from build123d import *

# Parameters (mm, degrees)
SALIENTE_EXTRUIR2_DEPTH      = 30.5
CROQUIS14_R                  = 25.5
CORTAR_EXTRUIR1_DEPTH        = 12
SALIENTE_EXTRUIR3_DEPTH      = 30
SALIENTE_EXTRUIR3_DEPTH_BACK = 4
CROQUIS15_R                  = 14
CROQUIS16_R                  = 11.5
CORTAR_EXTRUIR2_DEPTH        = 25
SKETCH1_W                    = 18
SKETCH1_H                    = 53
CUT_EXTRUDE1_DEPTH           = 8.5
SKETCH2_R                    = 4
CUT_EXTRUDE2_DEPTH           = 3
SKETCH3_R                    = 2.45
BOSS_EXTRUDE1_DEPTH          = 8.5
SKETCH4_W                    = 2.6
SKETCH4_H                    = 5
BOSS_EXTRUDE2_DEPTH          = 12.4


with BuildPart() as part:
    # Croquis13 → Saliente-Extruir2 (new body)
    with BuildSketch(Plane.XY):
        with BuildLine():
            Line((63.278452832, -47.557716663), (115.634697867, -47.557716663))
            add(Edge.make_bspline(
                [(115.634697867, -47.557716663), (120.956575349, -31.401681318), (120.956575349, -11.961207195)],
                knots=[0.980995561, 0.980995561, 0.980995561, 1.570796327, 1.570796327, 1.570796327], degree=2, weights=[1, 0.9568311, 1]))
            ThreePointArc((120.956575349, -11.961207195), (89.456575349, 19.538792805), (57.956575349, -11.961207195))
            add(Edge.make_bspline(
                [(57.956575349, -11.961207195), (57.956575349, -31.401681318), (63.278452832, -47.557716663)],
                knots=[4.71238898, 4.71238898, 4.71238898, 5.302189747, 5.302189747, 5.302189747], degree=2, weights=[1, 0.9568311, 1]))
        make_face()
    extrude(amount=SALIENTE_EXTRUIR2_DEPTH)

    # Croquis14 → Cortar-Extruir1 (cut)
    with BuildSketch(Plane.XY.offset(30.5)):
        with Locations((89.456575349, -11.961207195)):
            Circle(CROQUIS14_R)
        with BuildLine():
            add(Edge.make_bspline(
                [(109.141957532, -47.557716663), (114.956575349, -32.049805489), (114.956575349, -11.961207195)],
                knots=[4.023536226, 4.023536226, 4.023536226, 4.71238898, 4.71238898, 4.71238898], degree=2, weights=[1, 0.941269295, 1]))
            ThreePointArc((114.956575349, -11.961207195), (89.456575349, -37.461207195), (63.956575349, -11.961207195))
            add(Edge.make_bspline(
                [(63.956575349, -11.961207195), (63.956575349, -32.049805489), (69.771193166, -47.557716663)],
                knots=[1.570796327, 1.570796327, 1.570796327, 2.259649081, 2.259649081, 2.259649081], degree=2, weights=[1, 0.941269295, 1]))
            Line((69.771193166, -47.557716663), (109.141957532, -47.557716663))
        make_face()
    extrude(amount=-CORTAR_EXTRUIR1_DEPTH, mode=Mode.SUBTRACT)

    # Croquis15 → Saliente-Extruir3 (add, two sides: drawn at the far end of the back side and taken through both)
    with BuildSketch(Plane(origin=(89.456575349, 19.538792805, 30.5), x_dir=(1, 0, 0), z_dir=(0, 1, 0)).offset(-SALIENTE_EXTRUIR3_DEPTH_BACK)):
        with Locations(Location((0, 15.25, 0), (0, 0, 270))):
            Circle(CROQUIS15_R)
    extrude(amount=SALIENTE_EXTRUIR3_DEPTH + SALIENTE_EXTRUIR3_DEPTH_BACK)

    # Croquis16 → Cortar-Extruir2 (cut)
    with BuildSketch(Plane(origin=(0, 49.538792805, 0), x_dir=(1, 0, 0), z_dir=(0, 1, 0))):
        with Locations(Location((89.456575349, -15.25, 0), (0, 0, 270))):
            Circle(CROQUIS16_R)
    extrude(amount=-CORTAR_EXTRUIR2_DEPTH, mode=Mode.SUBTRACT)

    # Sketch1 → Cut-Extrude1 (cut)
    with BuildSketch(Plane(origin=(0, -29.057716663, 18.5), x_dir=(-1, 0, 0), z_dir=(0, 0, -1))):
        with Locations((-88.956575349, 11)):
            Rectangle(SKETCH1_W, SKETCH1_H)
    extrude(amount=CUT_EXTRUDE1_DEPTH, mode=Mode.SUBTRACT)

    # Sketch2 → Cut-Extrude2 (cut)
    with BuildSketch(Plane.XZ.offset(44.557716663)):
        with Locations((88.956575349, 18.5)):
            Circle(SKETCH2_R)
    extrude(amount=CUT_EXTRUDE2_DEPTH, mode=Mode.SUBTRACT)

    # Sketch3 → Boss-Extrude1 (add)
    with BuildSketch(Plane.XY.offset(18.5)):
        with Locations((104.956575349, -32.557716663)):
            Circle(SKETCH3_R)
        with Locations((104.956575349, -2.557716663)):
            Circle(SKETCH3_R)
        with Locations((70.956575349, -17.557716663)):
            Circle(SKETCH3_R)
        with Locations((106.956575349, -17.557716663)):
            Circle(SKETCH3_R)
        with Locations((72.956575349, -32.557716663)):
            Circle(SKETCH3_R)
        with Locations((72.956575349, -2.557716663)):
            Circle(SKETCH3_R)
    extrude(amount=BOSS_EXTRUDE1_DEPTH)

    # Sketch4 → Boss-Extrude2 (add)
    with BuildSketch(Plane.XY.offset(10)):
        with Locations((81.256575349, -8.257716663)):
            Rectangle(SKETCH4_W, SKETCH4_H)
        with Locations((96.656575349, -8.257716663)):
            Rectangle(SKETCH4_W, SKETCH4_H)
    extrude(amount=BOSS_EXTRUDE2_DEPTH)


solid = part.part
Source: CAD feature listing. Evaluate the final solid. Frame: model axes, mm. A direction names the side the tool comes from. Coordinates: 2 decimals unless noted, no trailing zeros. Loops run counter-clockwise (first coordinate to the right, second up) from the corner with the lowest first, then second, coordinate; pieces in that order, holes last. Notation, with made-up numbers: (80, -6) -> (90, -6) arc R31 cw to (90, 30) -> close; hole circle Ø10 at (19.5, 65.5). An arc over 180 degrees is marked (long way). Answer in a Markdown table with one row per item. Add a question column.
Q1. Section D-D on y = 26.5. Return the cut outline in (x, z).
Q2. Section B-B on z = 24. Give the number of separate pieces and of enclosed holes in the cut face, and give its area (3 significant figures).
Q3. Section A-A on x = 87.5. Return the cut outline in (y, z), and give its area (3 significant figures).
Q4. Section C-C on y = 4.5. Return the cut outline in (x, z).
Q5. Pull-direction query (Y, two-part tool) for faces 5 (the face through (100.878, 17.395, 4.87)), 6 (the face through (100.86, 37.21, 13.75)), 7 (the face through (89, -18, 10)), 8 (the face through (82.557, -8, 16)); classes: pulls with the +Y half, pulls with the -Y half, needs draft (parallel to the pull), parting line crosses it, or undercut.
Q6. Ray query, line 1 along Y through (x, z) = (82, 11); line 2 along X through (y, z) = (32.75, 15.25); line 3 along X through (y, z) = (-13, 21.5). Return the intervals inside material, ascending.
Q7. Contact query for flat-ended pins moving along their axis: pin 1 Ø4 at (x, y) = (86.5, 6) entering from +Z; pin 2 Ø2 at (x, y) = (97.5, -8.5) entering from +Z; pin 3 Ø4 at (y, z) = (36.5, 10) entering from -X; pin 4 Ø1.5 at (x, y) = (74, 14.5) entering from -Z. Output: stop coordinate, or through.
Q8. Reachability of faces 1 (the face through (89, -47.558, 12)), 2 (the face through (81, -8, 22.4)), 3 (the face through (71, -18, 27)), 4 (the face through (93.662, 32.665, 28.604)) from +Z, -Z, +X, -X, +Y, -Y: full face, straight path, thin tool, end or side. Return the list, or none.
Computed values:
| question | item | result |
|---|---|---|
| 1 | outline | circle Ø28 at (89.46, 15.25); hole circle Ø23 at (89.46, 15.25) |
| 2 | separate pieces | 7 |
| 2 | enclosed holes | 0 |
| 2 | area | 1,380 mm^2 |
| 3 | outline | (-47.56, 0) -> (19.48, 0) -> (19.48, 1.39) -> (49.54, 1.39) -> (49.54, 3.92) -> (24.54, 3.92) -> (24.54, 26.58) -> (49.54, 26.58) -> (49.54, 29.11) -> (19.48, 29.11) -> (19.48, 30.5) -> (13.46, 30.5) -> (13.46, 18.5) -> (8.44, 18.5) -> (8.44, 10) -> (-44.56, 10) -> (-44.56, 14.77) -> (-47.56, 14.77) -> close |
| 3 | area | 1,120 mm^2 |
| 4 | outline | (62.6, 0) -> (116.31, 0) -> (116.31, 30.5) -> (108.93, 30.5) -> (108.93, 18.5) -> (97.96, 18.5) -> (97.96, 10) -> (79.96, 10) -> (79.96, 18.5) -> (69.98, 18.5) -> (69.98, 30.5) -> (62.6, 30.5) -> close |
| 5 | face 5 | pulls with the +Y half |
| 5 | face 6 | needs draft |
| 5 | face 7 | undercut |
| 5 | face 8 | undercut |
| 6 | line 1 | y = -47.56 to -44.56, -10.76 to -5.76, 8.44 to 24.54 |
| 6 | line 2 | x = 75.46 to 77.96, 100.96 to 103.46 |
| 6 | line 3 | x = 57.96 to 63.96, 114.95 to 120.95 |
| 7 | pin 1 | stops at z = 10 |
| 7 | pin 2 | stops at z = 22.4 |
| 7 | pin 3 | stops at x = 75.84 |
| 7 | pin 4 | stops at z = 0 |
| 8 | face 1 | +Z, -Z, +X, -X, -Y |
| 8 | face 2 | +Z, -Y |
| 8 | face 3 | +Z |
| 8 | face 4 | +Y |
